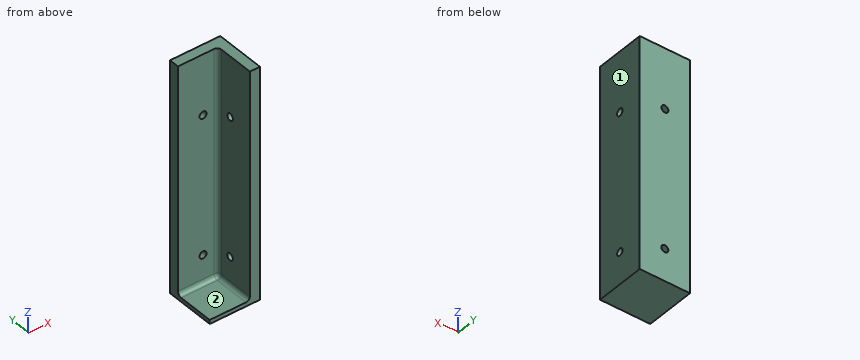
Autodesk Inventor part; units mm, degrees
ref_plane "YZ Plane" through (0, 0, 0) normal (1, 0, 0) x (0, 1, 0)
ref_plane "XZ Plane" through (0, 0, 0) normal (0, 1, 0) x (-1, 0, 0)
ref_plane "XY Plane" through (0, 0, 0) normal (0, 0, 1) x (1, 0, 0)
sketch "Sketch1" plane through (0, 0, 0) normal (0, 1, 0) x (-1, 0, 0)
  line L0 (0, 0) -> (0, 115)
  line L1 (0, 115) -> (5, 115)
  line L2 (0, 0) -> (25, 0)
  line L3 (25, 0) -> (25, 2)
  line L4 (5, 115) -> (5, 0)
  line L5 (25, 2) -> (0, 2)
  line L6 (5, 2) -> (10, 2)
  line L7 (5, 7) -> (5, 2)
  dimension "d1" = 5
  dimension "d2" = 25
  dimension "d3" = 2
  dimension "d60" = 115
extrude "Extrusion2" add sketch "Sketch1" along normal blind 20
sketch "Sketch3" plane through (0, 20, 0) normal (0, 1, 0) x (1, 0, 0)
  line L0 (0, 0) -> (-25, 0)
  line L1 (-25, 0) -> (-25, -2)
  line L2 (-25, 0) -> (-25, -2)
  line L3 (-25, -2) -> (-5, -2)
  line L4 (-5, -115) -> (0, -115)
  line L5 (-5, -115) -> (0, -115)
  line L6 (0, 0) -> (-25, 0)
  line L7 (0, -115) -> (0, 0)
  line L8 (-5, -115) -> (-25, -115)
  line L9 (-25, -115) -> (-25, -2)
extrude "Extrusion3" add sketch "Sketch3" along normal blind 5
fillet "Face Fillet1" radius 2 1 edges at (-5, 10, 2)
fillet "Face Fillet2" radius 2 1 edges at (-16, 20, 2)
hole "Hole3" at (0, 12.5, 15.9996) direction (-1, 0, 0) diameter 3.5 depth 8.8
hole "Hole4" at (-12.5, 25, 16) direction (0, -1, 0) diameter 3.5 depth 8.8
sketch "Sketch11" plane through (0, 25, 0) normal (0, 1, 0) x (1, 0, 0)
  line L0 (-5, -115) -> (0, -115)
  line L1 (0, -115) -> (-12.5, -115)
  line L2 (-12.5, -115) -> (-12.5, -85)
  line L3 (-12.5, -85) -> (0, -85)
  line L4 (0, -85) -> (0, -115)
  point P0 (0, 0)
  dimension "d82" = 12.5
  dimension "d83" = 30
hole "Hole7" at (-12.5, 25, 85) direction (0, -1, 0) diameter 3.5 depth 8.8
sketch "Sketch12" plane through (0, 0, 115) normal (1, 0, 0) x (0, 0, -1)
  line L0 (115, 25) -> (0, 25)
  line L1 (0, 25) -> (30, 25)
  line L2 (30, 25) -> (30, 12.5)
  line L3 (30, 12.5) -> (0, 12.5)
  line L4 (0, 12.5) -> (0, 25)
  point P0 (115, 0)
  dimension "d91" = 30
  dimension "d92" = 12.5
hole "Hole8" at (0, 12.5, 85) direction (-1, 0, 0) diameter 3.5 depth 8.8
properties part number "wall-joint"
Design review of the part built by this model. Coordinates are the model's own, in mm. Face numbers are marked on the shaded views. A direction names the side the tool comes from. Give positions to 0.01 mm unless a question says otherwise; leave off trailing zeros. Order: outer loops, then holes, each group sorted by start corner. A loop starts at its lowest first (then second) coordinate and runs counter-clockwise, first axis right, second up. Notation, with made-up numbers: (-33, 47) - (-14, 47) arc R25 ccw to (-14, 85) - close; hole circle Ø10 at (-21.75, -4.75). An arc over 180 degrees is marked (long way). Use a Markdown table: item, result. Add a question column.
(1) Add section C-C on y = 7.25. Give the boundary of the cut face in (x, z).
(2) Machinability: for the marked faces 1 and 2, which of the approach directions +Z, -Z, +X, -X, +Y, -Y give a long, thin tool a straight path to every point of the face, cutting with its end or side? Answer none if there is none.
(3) Add section D-D on x = -6. Give the boundary of the cut face in (y, z), then the cut area to 3 significant figures.
(4) Clearance check with flat-ended pins moving along their axes: P1, Ø3, axis at y = 8, z = 54, coming from the -X side; P2, Ø1, axis at x = -21.5, y = 13, coming from the +Z side; P3, Ø9, axis at x = -18.5, z = 39.5, coming from the -Y side. State where each tip first meets the part, or that it passes through.
(5) Add section A-A on z = 85. Give the boundary of the cut face in (x, y).
(6) Wall thickness on probe 1 along Z at (x, y) = (-1.25, 12.5); probe 2 along X at (y, z) = (23.5, 85): over which ranges is each line inside the solid? List them lowest first. Write a range as [from, to].
(7) Add section B-B on x = -12.5. Give the boundary of the cut face in (y, z), then the cut area to 3 significant figures.
Report:
| question | item | result |
|---|---|---|
| 1 | outline | (-25, 0) - (0, 0) - (0, 115) - (-5, 115) - (-5, 4) arc R2 cw to (-7, 2) - (-25, 2) - close |
| 2 | face 1 | +Z, -Z, +X, +Y, -Y |
| 2 | face 2 | +Z, -X, -Y |
| 3 | outline | (0, 0) - (25, 0) - (25, 115) - (19.73, 115) - (19.73, 4) arc R1.73 cw to (18, 2.27) - (0, 2.27) - close |
| 3 | area | 651 mm² |
| 4 | P1 | stops at x = -5 |
| 4 | P2 | stops at z = 2 |
| 4 | P3 | stops at y = 20 |
| 5 | outline | (-25, 20) - (-14.25, 20) - (-14.25, 25) - (-25, 25) - close; (-10.75, 20) - (-7, 20) arc R2 cw to (-5, 18) - (-5, 14.25) - (0, 14.25) - (0, 25) - (-10.75, 25) - close; (-5, 0) - (0, 0) - (0, 10.75) - (-5, 10.75) - close |
| 6 | probe 1 | z = [0, 14.25], [17.75, 83.25], [86.75, 115] |
| 6 | probe 2 | x = [-25, -14.25], [-10.75, 0] |
| 7 | outline | (0, 0) - (25, 0) - (25, 14.25) - (20, 14.25) - (20, 4) arc R2 cw to (18, 2) - (0, 2) - close; (20, 17.75) - (25, 17.75) - (25, 83.25) - (20, 83.25) - close; (20, 86.75) - (25, 86.75) - (25, 115) - (20, 115) - close |
| 7 | area | 581 mm² |
